Part model, mm, in its own coordinate system. Face numbers are marked on the shaded views. Coordinates: 2 decimals unless noted, no trailing zeros. Write each loop counter-clockwise with the first axis right and the second up, starting at its lowest first coordinate (ties: lowest second). Pieces come first, ordered by that corner, then holes. Notation, with made-up numbers: (87.25, -11.75) - (112.25, -11.75) arc R16 ccw to (112.25, -2.75) - close; hole circle Ø10 at (29, 84). An arc over 180 degrees is marked (long way). Write each question's results on one line, items separated by ' | '.
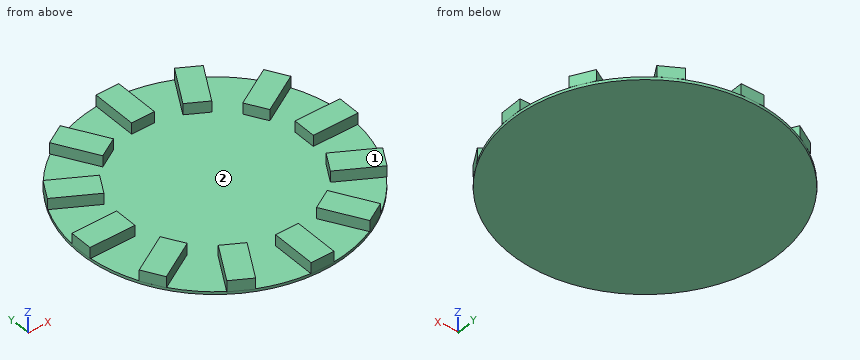
from build123d import *

# Parameters (mm, degrees)
F0_W     = 25.849619
F0_H     = 50.748426
F0_W_2   = 50.748426
F0_H_2   = 25.849619
F1_DEPTH = 12.7
F2_R     = 152.4
F3_DEPTH = 3.175


with BuildPart() as f1:
    # F0 (on Top) → F1 (new body)
    with BuildSketch(Plane.XY):
        with Locations((-0.551344, 127)):
            Rectangle(F0_W, F0_H)
        Polygon((-40.097159, 94.197246), (-65.471372, 138.146671), (-87.857798, 125.221862), (-62.483585, 81.272437), align=None)
        Polygon((-81.823781, 61.528628), (-125.773207, 86.902841), (-138.698016, 64.516415), (-94.748591, 39.142202), align=None)
        with Locations((-127, -0.551344)):
            Rectangle(F0_W_2, F0_H_2)
        Polygon((-94.197246, -40.097159), (-138.146671, -65.471372), (-125.221862, -87.857798), (-81.272437, -62.483585), align=None)
        Polygon((-61.528628, -81.823781), (-86.902841, -125.773207), (-64.516415, -138.698016), (-39.142202, -94.748591), align=None)
        with Locations((0.551344, -127)):
            Rectangle(F0_W, F0_H)
        Polygon((40.097159, -94.197246), (65.471372, -138.146671), (87.857798, -125.221862), (62.483585, -81.272437), align=None)
        Polygon((81.823781, -61.528628), (125.773207, -86.902841), (138.698016, -64.516415), (94.748591, -39.142202), align=None)
        with Locations((127, 0.551344)):
            Rectangle(F0_W_2, F0_H_2)
        Polygon((94.197246, 40.097159), (138.146671, 65.471372), (125.221862, 87.857798), (81.272437, 62.483585), align=None)
        Polygon((61.528628, 81.823781), (86.902841, 125.773207), (64.516415, 138.698016), (39.142202, 94.748591), align=None)
    extrude(amount=F1_DEPTH)

    # F2 (on Top) → F3 (join)
    with BuildSketch(Plane.XY):
        Circle(F2_R)
    extrude(amount=-F3_DEPTH)


solid = f1.part
(1) Saw through at B-B on z = 2.5. Count the separate pieces of the cut face and the enclosed holes in it, then the cut area to 3 significant figures.
Return value:
separate pieces: 12 | enclosed holes: 0 | area: 15,700 mm^2
(2) Saw through at A-A on y = 51.5. Write the cut outline in (x, z) (3 decimals).
Return value:
outline: (-143.435, -3.175) - (143.435, -3.175) - (143.435, 0) - (113.948, 0) - (113.948, 12.7) - (87.614, 12.7) - (87.614, 0) - (-87.614, 0) - (-87.614, 12.7) - (-116.153, 12.7) - (-116.153, 0) - (-143.435, 0) - close
(3) Saw through at C-C on y = -33.5. Write the cut outline in (x, z) (1 decimal).
Return value:
outline: (-148.7, -3.2) - (148.7, -3.2) - (148.7, 0) - (-148.7, 0) - close
(4) Flat gauge pins, fed straight in: P1, Ø5.5, axis at x = 84.5, y = 129, coming from the -Z side (3 decimals); P2, Ø4, axis at x = 37.5, y = -26, coming from the +Z side; P3, Ø4, axis at y = 87.5, z = 1, coming from the -X side; P4, Ø8, axis at x = -28, z = 2.5, coming from the +Y side. Where does each tip first touch, or does it go through?
Return value:
P1: stops at z = -3.175 | P2: stops at z = 0 | P3: stops at x = -126.58 | P4: stops at y = 150.36
(5) Wall check: line 1 (X direction, y = 121, z = 4.75); line 2 (X direction, y = -7.5, z = 3.25); line 3 (X direction, y = -130, z = 0.25). Give the ranges that are in metal, low to high. Write a range as from..to.
Return value:
line 1: x = -85.42..-55.57, -13.48..12.37, 54.3..84.15 | line 2: x = -152.37..-101.63, 101.63..152.37 | line 3: x = -79.58..-59.49, -12.37..13.48, 60.77..79.58
(6) Two-plate mould, pull along Y, no slides. Class the marked faces 1 and 2: released by +Y, released by -Y, zero draft, split by the parting line, or undercut.
Return value:
face 1: zero draft | face 2: undercut
